Work out the finished part from the listing and answer in its coordinate system (mm). Face numbers are marked on the shaded views. A direction names the side the tool comes from. Round coordinates to 2 decimals unless told otherwise and drop trailing zeros. Write each loop counter-clockwise with the first axis right and the second up, starting at its lowest first coordinate (ties: lowest second). Pieces come first, ordered by that corner, then holes. Notation, with made-up numbers: M 46.25,-32.5 L 57.25,-32.5 A10 cw 57.25,-20.5 Z; hole C 55.5,18 d11. An arc over 180 degrees is marked long. One line per item, written item: value. Start each with the question number.
Q1. A tool of negligible diameter and unlimited length cuts with its end or side. For the marked faces 4, 5 and 6, from which of +Z, -Z, +X, -X, +Y, -Y can it reach the whole face along a straight path? Write none if from no direction.
Q2. Find section C-C (y = 1.75). Write down the section's boundary in (x, z) (3 decimals), and give its area (3 significant figures).
Q3. Find section A-A (x = -6.35). Write down the section's boundary in (y, z) (3 decimals).
Q4. Given pin 1 Ø2 at (x, y) = (4.5, 4.5) entering from +Z; pin 2 Ø3 at (y, z) = (5, 5.5) entering from +X (3 decimals); pin 3 Ø3 at (x, z) = (-6.5, 4.5) entering from +Y (3 decimals), each flat-ended and moving along its own axis, determine where each tip first touches the part or whether it passes through.
Q5. Consider probe 1 along Y at (x, z) = (0, 2.75) (1 decimal); probe 2 along Z at (x, y) = (-6.35, -0.5); probe 3 along X at (y, z) = (1, 4) (3 decimals). Determine where each line is inside the solid, lowest interval first.
Q6. Find section B-B (z = 2.5). Write down the section's boundary in (x, y) (1 decimal), and give its area (3 significant figures).
Q7. The mould has two halves that part along X. Classify the marked faces 1, 2 and 3: released by +X, released by -X, zero draft, split by the parting line, or undercut.
from build123d import *

# Parameters (mm, degrees)
SKETCH1_W                        = 19.05
SKETCH1_H                        = 6.35
BOSS_EXTRUDE1_DEPTH              = 6.35
SKETCH6_W                        = 6.35
SKETCH6_H                        = 6.35
BOSS_EXTRUDE2_DEPTH              = 4.7625
TAPPED_HOLE_FOR_4_40_HELICOIL1_D = 3.048
TAPPED_HOLE_FOR_4_40_HELICOIL2_D = 3.048


with BuildPart() as part:
    # Sketch1 → Boss-Extrude1 (new body)
    with BuildSketch(Plane.XY):
        Rectangle(SKETCH1_W, SKETCH1_H)
    extrude(amount=BOSS_EXTRUDE1_DEPTH)

    # Sketch6 → Boss-Extrude2 (add)
    with BuildSketch(Plane(origin=(0, 3.175, 0), x_dir=(1, 0, 0), z_dir=(0, 1, 0))):
        with Locations((0, -3.175)):
            Rectangle(SKETCH6_W, SKETCH6_H)
    extrude(amount=BOSS_EXTRUDE2_DEPTH)

    # Tapped Hole for #4-40 Helicoil1 (through all)
    with Locations(Plane(origin=(0, 3.175, 0), x_dir=(1, 0, 0), z_dir=(0, 1, 0))):
        with Locations((-6.35, -3.175), (6.35, -3.175)):
            Hole(TAPPED_HOLE_FOR_4_40_HELICOIL1_D / 2)

    # Tapped Hole for #4-40 Helicoil2 (through all)
    with Locations(Plane.XY.offset(6.35)):
        with Locations((0, 4.7625)):
            Hole(TAPPED_HOLE_FOR_4_40_HELICOIL2_D / 2)


solid = part.part
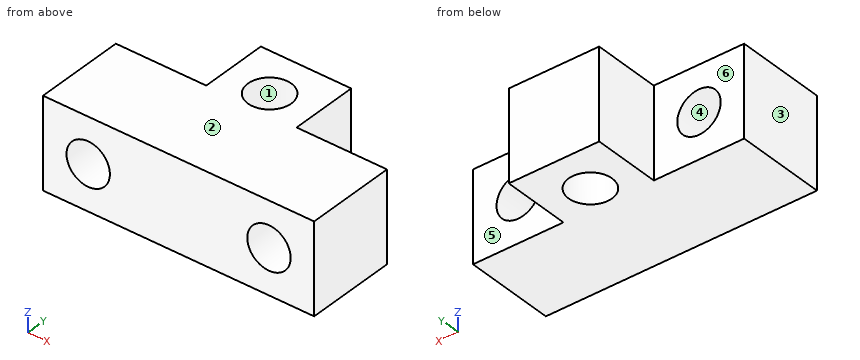
The answers:
1. face 4: +Y, -Y
1. face 5: +Z, -Z, +X, +Y
1. face 6: +Z, -Z, -X, +Y
2. outline: M -9.525,0 L 9.525,0 L 9.525,6.35 L -9.525,6.35 Z; hole C -6.35,3.175 d3.048; hole C 6.35,3.175 d3.048
2. area: 106 mm2
3. outline: M -3.175,0 L 3.175,0 L 3.175,1.651 L -3.175,1.651 Z; M -3.175,4.699 L 3.175,4.699 L 3.175,6.35 L -3.175,6.35 Z
4. pin 1: through
4. pin 2: x = 3.175
4. pin 3: y = 3.175
5. probe 1: -3.2 to 3.2, 6.3 to 7.9
5. probe 2: 0 to 1.65, 4.7 to 6.35
5. probe 3: -9.525 to -7.631, -5.069 to 5.069, 7.631 to 9.525
6. outline: M -9.5,-3.2 L -7.7,-3.2 L -7.7,3.2 L -9.5,3.2 Z; M -5,-3.2 L 5,-3.2 L 5,3.2 L 3.2,3.2 L 3.2,7.9 L -3.2,7.9 L -3.2,3.2 L -5,3.2 Z; M 7.7,-3.2 L 9.5,-3.2 L 9.5,3.2 L 7.7,3.2 Z; hole C 0,4.8 d3
6. area: 109 mm2
7. face 1: undercut
7. face 2: zero draft
7. face 3: released by -X
